The figure shows three views and two pictorial views of one solid part (mm, origin at its lowest corner). Answer the questions. Coordinates: 2 decimals unless noted, no trailing zeros. Order: outer loops, then holes, each group sorted by start corner. A loop starts at its lowest first (then second) coordinate and runs counter-clockwise, first axis right, second up. Notation, with made-up numbers: (49, 40) -> (75, 40) arc R20 cw to (75, 74) -> close; hole circle Ø11 at (44, 28). An arc over 180 degrees is marked (long way). Write item = value, one per line.
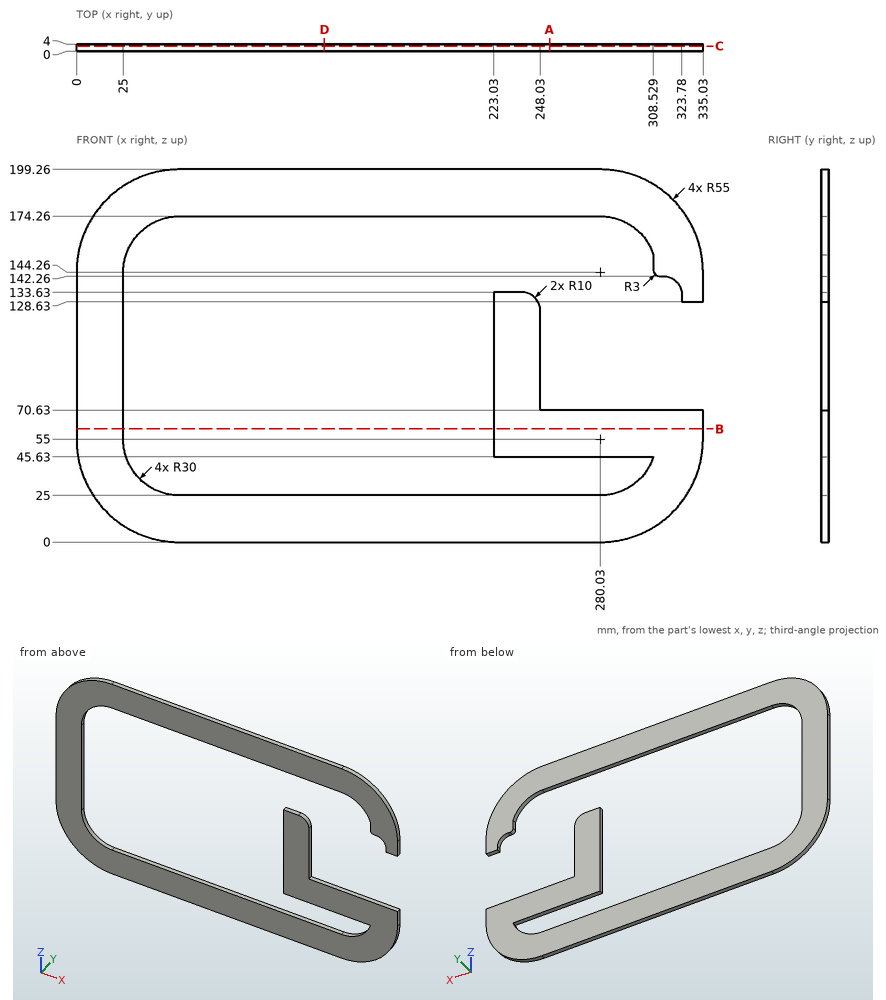
Q1. Section C-C, the plane y = 2.8 is taken. Give the vertices of the cut face in (x, z).
The answers:
outline = (0, 55) arc R55 ccw to (55, 0) -> (280.03, 0) arc R55 ccw to (335.03, 55) -> (335.03, 70.63) -> (248.03, 70.63) -> (248.03, 123.63) arc R10 ccw to (238.03, 133.63) -> (223.03, 133.63) -> (223.03, 45.63) -> (308.53, 45.63) arc R30 cw to (280.03, 25) -> (55, 25) arc R30 cw to (25, 55) -> (25, 144.26) arc R30 cw to (55, 174.26) -> (280.03, 174.26) arc R30 cw to (308.53, 153.63) -> (308.53, 145.26) arc R3 ccw to (311.53, 142.26) -> (313.78, 142.26) arc R10 cw to (323.78, 132.26) -> (323.78, 128.63) -> (335.03, 128.63) -> (335.03, 144.26) arc R55 ccw to (280.03, 199.26) -> (55, 199.26) arc R55 ccw to (0, 144.26) -> close
Q2. Section A-A, the plane x = 253 is taken. Give the vertices of the cut face in (y, z).
The answers:
outline = (0, 0) -> (4, 0) -> (4, 25) -> (0, 25) -> close; (0, 45.63) -> (4, 45.63) -> (4, 70.63) -> (0, 70.63) -> close; (0, 174.26) -> (4, 174.26) -> (4, 199.26) -> (0, 199.26) -> close
Q3. Each of these flat-tipped pins is pushed along its axis until it touches: pin 1 Ø0.7 at (x, y) = (313, 2.5) entering from -Z; pin 2 Ø1.2 at (y, z) = (2, 151) entering from -X. Where does it stop, or does it pass through?
The answers:
pin_1 = 10.72
pin_2 = 0.34
Q4. Section D-D, the plane x = 132.5 is taken. Give the vertices of the cut face in (y, z), plus the area to 3 significant figures.
The answers:
outline = (0, 0) -> (4, 0) -> (4, 25) -> (0, 25) -> close; (0, 174.26) -> (4, 174.26) -> (4, 199.26) -> (0, 199.26) -> close
area = 200 mm2
Q5. Section B-B, the plane z = 60.5 is taken. Give the vertices of the cut face in (x, y), plus the area to 3 significant figures.
The answers:
outline = (0, 0) -> (25, 0) -> (25, 4) -> (0, 4) -> close; (223.03, 0) -> (335.03, 0) -> (335.03, 4) -> (223.03, 4) -> close
area = 548 mm2
Q6. Find the intervals of material crossed by line 1 along Z through (x, y) = (260, 3.25); line 2 along Z through (x, y) = (161, 0.2); line 3 along X through (y, z) = (2.7, 55.5), in increasing order.
The answers:
line_1 = 0 to 25, 45.63 to 70.63, 174.26 to 199.26
line_2 = 0 to 25, 174.26 to 199.26
line_3 = 0 to 25, 223.03 to 335.03
